Autodesk Inventor part; units mm, degrees
ref_plane "YZ Plane" through (0, 0, 0) normal (1, 0, 0) x (0, 1, 0)
ref_plane "XZ Plane" through (0, 0, 0) normal (0, 1, 0) x (-1, 0, 0)
ref_plane "XY Plane" through (0, 0, 0) normal (0, 0, 1) x (1, 0, 0)
sketch "Sketch1" plane through (0, 0, 0) normal (0, 0, 1) x (1, 0, 0)
  circle A0 centre (0, 0) radius 16.5
  dimension "d0" = 33
extrude "Body" add sketch "Sketch1" along normal blind 9
sketch "Sketch2" plane through (0, 0, 9) normal (0, 0, 1) x (1, 0, 0)
  circle A0 centre (0, 0) radius 16.5
  circle A1 centre (0, 0) radius 6
  line L0 (-6, 0) -> (-6, -15.3704)
  line L1 (6, 0) -> (6, -15.3704)
  arc A2 (-6, -15.3704) -> (6, -15.3704) centre (0, 0) ccw
  dimension "d3" = 12
extrude "Main Cutout" cut sketch "Sketch2" against normal blind 9 contours L0 A1 L1 A0 | A1 picked at (0.2411, -12.9009)
sketch "Sketch4" plane through (0, 0, 9) normal (0, 0, 1) x (1, 0, 0)
  line L0 (6, 0) -> (6, -15.3704)
  arc A0 (6, -15.3704) -> (-6, -15.3704) centre (0, 0) ccw
  line L1 (-6, -15.3704) -> (-6, 0)
  arc A1 (6, 0) -> (-6, 0) centre (0, 0) ccw
  circle A2 centre (0, 0) radius 8
  line L2 (-8, 0) -> (-8, -14.4309)
  line L3 (8, 0) -> (8, -14.4309)
  arc A3 (-8, -14.4309) -> (8, -14.4309) centre (0, 0) ccw
  dimension "d7" = 16
extrude "Bottom Cutout" cut sketch "Sketch4" against normal blind 3.2 contours A1 L1 A2 L0 | A2 L3 A0 L0 | L1 A0 L2 A2 picked at (-6.3631, -2.9996)
sketch "Sketch7" plane through (0, 0, 0) normal (0, 0, -1) x (-1, 0, 0)
  arc A0 (6, 0) -> (-6, 0) centre (0, 0) ccw
  arc A1 (6, -15.3704) -> (-6, -15.3704) centre (0, 0) ccw
  circle A2 centre (0, 0) radius 12.5 construction
  circle A3 centre (0, 12.5) radius 1.6
  circle A4 centre (-10.8253, 6.25) radius 1.6
  circle A5 centre (-10.8253, -6.25) radius 1.6
  circle A6 centre (0, -12.5) radius 1.6
  circle A7 centre (10.8253, -6.25) radius 1.6
  circle A8 centre (10.8253, 6.25) radius 1.6
  dimension "d18" = 25
  dimension "d19" = 3.2
  dimension "d22" = 360
extrude "M3 Holes" cut sketch "Sketch7" against normal blind 7 contours A3 | A4 | A5 | A7 | A8
sketch "Sketch8" plane through (0, 0, 9) normal (0, 0, 1) x (1, 0, 0)
  arc A0 (8, 0) -> (-8, 0) centre (0, 0) ccw
  circle A1 centre (0, 0) radius 12.5 construction
  circle A2 centre (0, 12.5) radius 1.5 construction
  circle A3 centre (-10.8253, 6.25) radius 1.5 construction
  circle A4 centre (-10.8253, -6.25) radius 1.5 construction
  circle A5 centre (0, -12.5) radius 1.5 construction
  circle A6 centre (10.8253, -6.25) radius 1.5 construction
  circle A7 centre (10.8253, 6.25) radius 1.5 construction
  line L0 (0, 9.238) -> (-2.825, 10.869)
  line L1 (-2.825, 10.869) -> (-2.825, 14.131)
  line L2 (-2.825, 14.131) -> (0, 15.762)
  line L3 (0, 15.762) -> (2.825, 14.131)
  line L4 (2.825, 14.131) -> (2.825, 10.869)
  line L5 (2.825, 10.869) -> (0, 9.238)
  line L6 (-10.8253, 2.988) -> (-13.6503, 4.619)
  line L7 (-13.6503, 4.619) -> (-13.6503, 7.881)
  line L8 (-13.6503, 7.881) -> (-10.8253, 9.512)
  line L9 (-10.8253, 9.512) -> (-8.0003, 7.881)
  line L10 (-8.0003, 7.881) -> (-8.0003, 4.619)
  line L11 (-8.0003, 4.619) -> (-10.8253, 2.988)
  line L12 (10.8253, 2.988) -> (8.0003, 4.619)
  line L13 (8.0003, 4.619) -> (8.0003, 7.881)
  line L14 (8.0003, 7.881) -> (10.8253, 9.512)
  line L15 (10.8253, 9.512) -> (13.6503, 7.881)
  line L16 (13.6503, 7.881) -> (13.6503, 4.619)
  line L17 (13.6503, 4.619) -> (10.8253, 2.988)
  line L18 (-10.8253, -9.5178) -> (-13.6553, -7.8839)
  line L19 (-13.6553, -7.8839) -> (-13.6553, -4.6161)
  line L20 (-13.6553, -4.6161) -> (-10.8253, -2.9822)
  line L21 (-10.8253, -2.9822) -> (-7.9953, -4.6161)
  line L22 (-7.9953, -4.6161) -> (-7.9953, -7.8839)
  line L23 (-7.9953, -7.8839) -> (-10.8253, -9.5178)
  line L24 (10.8253, -9.5178) -> (7.9953, -7.8839)
  line L25 (7.9953, -7.8839) -> (7.9953, -4.6161)
  line L26 (7.9953, -4.6161) -> (10.8253, -2.9822)
  line L27 (10.8253, -2.9822) -> (13.6553, -4.6161)
  line L28 (13.6553, -4.6161) -> (13.6553, -7.8839)
  line L29 (13.6553, -7.8839) -> (10.8253, -9.5178)
  dimension "d26" = 25
  dimension "d27" = 3
  dimension "d30" = 360
  dimension "d32" = 5.65
  dimension "d33" = 5.65
  dimension "d34" = 5.65
  dimension "d35" = 5.66
  dimension "d36" = 5.66
extrude "M3 Nut Traps" cut sketch "Sketch8" against normal blind 3.2
sketch "Sketch9" plane through (0, 0, 9) normal (0, 0, 1) x (1, 0, 0)
  line L0 (-8, -7.8866) -> (-10.8253, -9.5178)
  line L1 (-10.8253, -9.5178) -> (-13.6553, -7.8839)
  line L2 (-13.6553, -7.8839) -> (-13.6553, -4.6161)
  line L3 (-13.6553, -4.6161) -> (-10.8253, -2.9822)
  line L4 (-10.8253, -2.9822) -> (-8, -4.6134)
  line L5 (-8, -4.6134) -> (-8, 0)
  arc A0 (8, 0) -> (-8, 0) centre (0, 0) ccw
  line L6 (8, 0) -> (8, -4.6134)
  line L7 (8, -4.6134) -> (10.8253, -2.9822)
  line L8 (10.8253, -2.9822) -> (13.6553, -4.6161)
  line L9 (13.6553, -4.6161) -> (13.6553, -7.8839)
  line L10 (13.6553, -7.8839) -> (10.8253, -9.5178)
  line L11 (10.8253, -9.5178) -> (8, -7.8866)
  line L12 (8, -7.8866) -> (8, -14.4309)
  arc A1 (8, -14.4309) -> (-8, -14.4309) centre (0, 0) ccw
  line L13 (-8, -14.4309) -> (-8, -7.8866)
  line L14 (13.6503, 4.619) -> (10.8253, 2.988)
  line L15 (10.8253, 2.988) -> (8.0003, 4.619)
  line L16 (8.0003, 4.619) -> (8.0003, 7.881)
  line L17 (8.0003, 7.881) -> (10.8253, 9.512)
  line L18 (10.8253, 9.512) -> (13.6503, 7.881)
  line L19 (13.6503, 7.881) -> (13.6503, 4.619)
  line L20 (2.825, 10.869) -> (0, 9.238)
  line L21 (0, 9.238) -> (-2.825, 10.869)
  line L22 (-2.825, 10.869) -> (-2.825, 14.131)
  line L23 (-2.825, 14.131) -> (0, 15.762)
  line L24 (0, 15.762) -> (2.825, 14.131)
  line L25 (2.825, 14.131) -> (2.825, 10.869)
  line L26 (-8.0003, 4.619) -> (-10.8253, 2.988)
  line L27 (-10.8253, 2.988) -> (-13.6503, 4.619)
  line L28 (-13.6503, 4.619) -> (-13.6503, 7.881)
  line L29 (-13.6503, 7.881) -> (-10.8253, 9.512)
  line L30 (-10.8253, 9.512) -> (-8.0003, 7.881)
  line L31 (-8.0003, 7.881) -> (-8.0003, 4.619)
properties part number "Kossel E3D V6 Mount"
Check sheet for the modelled part. Datum: model origin and axes. Units: mm. A direction names the side the tool comes from. Coordinates: 2 decimals unless noted, no trailing zeros. Loops run counter-clockwise (first coordinate to the right, second up) from the corner with the lowest first, then second, coordinate; pieces in that order, holes last.
1) Sectioned sample at B-B (y = 4). Record the boundary of the cut face in (x, z), and give its area (3 significant figures).
2) Access from +Z, -Z, +X, -X, +Y, -Y to the whole of each face (thin tool, end or side, straight path). Record for faces 1 (the face through (-8, -11, 7)), 2 (the face through (9.433, 3.792, 7.422)), 3 (the face through (6, -8, 3)), 4 (the face through (-9.556, 5.276, 2.859)).
3) Sectioned sample at C-C (x = 1). Record the boundary of the cut face in (y, z), and give its area (3 significant figures).
4) Sectioned sample at D-D (z = 8). Count the separate pieces of the cut face and the enclosed holes in it, and give its area (3 significant figures).
5) Gauge pin test, flat ends, axial feed: pin 1 (1.5 mm diameter, centred on x = 5.5, y = -0.5, fed in from +Z); pin 2 (1.7 mm diameter, centred on y = -5.5, z = 2.5, fed in from +X); pin 3 (1.5 mm diameter, centred on x = -10.5, z = 1, fed in from +Y). Record the tip position at first contact, or that the pin passes through.
6) Sectioned sample at A-A (z = 1.75). Record the boundary of the cut face in (x, y), and give its area (3 significant figures).
7) Material ranges on probe 1 along X at (y, z) = (9, 8); probe 2 along Y at (x, z) = (11, 1); probe 3 along Y at (x, z) = (13, 6.25), recorded low to high.
Check sheet entries:
1. outline: (-16.01, 0) - (-4.47, 0) - (-4.47, 5.8) - (-6.93, 5.8) - (-6.93, 9) - (-9.07, 9) - (-9.07, 5.8) - (-12.58, 5.8) - (-12.58, 9) - (-16.01, 9) - close; (4.47, 0) - (16.01, 0) - (16.01, 9) - (12.58, 9) - (12.58, 5.8) - (9.07, 5.8) - (9.07, 9) - (6.93, 9) - (6.93, 5.8) - (4.47, 5.8) - close
1. area: 169 mm2
2. face 1: +Z, -Y
2. face 2: +Z
2. face 3: +Z, -Z, -Y
2. face 4: +Z, -Z
3. outline: (5.92, 0) - (11.25, 0) - (11.25, 5.8) - (9.82, 5.8) - (9.82, 9) - (7.94, 9) - (7.94, 5.8) - (5.92, 5.8) - close; (13.75, 0) - (16.47, 0) - (16.47, 9) - (15.18, 9) - (15.18, 5.8) - (13.75, 5.8) - close
3. area: 56.8 mm2
4. separate pieces: 1
4. enclosed holes: 3
4. area: 363 mm2
5. pin 1: stops at z = 5.8
5. pin 2: stops at x = 15.83
5. pin 3: stops at y = 13.31
6. outline: (-6, -15.37) - (-6, 0) arc R6 cw to (6, 0) - (6, -15.37) arc R16.5 ccw (long way) to start; hole circle Ø3.2 at (-10.83, -6.25); hole circle Ø3.2 at (-10.83, 6.25); hole circle Ø3.2 at (0, 12.5); hole circle Ø3.2 at (10.83, -6.25); hole circle Ø3.2 at (10.83, 6.25)
6. area: 565 mm2
7. probe 1: x = -13.83 to -11.71, -9.94 to 9.94, 11.71 to 13.83
7. probe 2: y = -12.3 to -7.84, -4.66 to 4.66, 7.84 to 12.3
7. probe 3: y = -10.16 to -8.26, -4.24 to 4.24, 8.26 to 10.16
